from build123d import *

# Parameters (mm, degrees)
F0_W          = 152.4
F0_H          = 203.2
F1_DEPTH      = 6.35
F3_DEPTH      = 63.5
F4_T          = 5
F4_T3_DEPTH   = 73.5
F4_T5_DEPTH   = 137
F6_R          = 13.716
F7_DEPTH      = 76.2
F5_W          = 101.6
F5_H          = 20
F8_DEPTH      = 63.501
F8_DEPTH_BACK = 139.701
F10_DEPTH     = 71.337


# Not quite as in the source:
# - a shell that OpenCascade refuses in one call is made with other operations: the cavity is built on its own and cut out


with BuildPart() as f1:
    # F0 (on Top) → F1 (new body)
    with BuildSketch(Plane.XY):
        Rectangle(F0_W, F0_H)
    extrude(amount=-F1_DEPTH)

    # F2 (on Right) → F3 (join, symmetric)
    with BuildSketch(Plane.YZ):
        Polygon((-101.6, 60), (-101.6, 0), (-38.1, 0), (-38.1, 20), (-68.58, 60), align=None)
    extrude(amount=F3_DEPTH, both=True)

    # F4: shell of thickness 5, made by hand


with BuildPart() as f4_core1:
    # F4_t2: copy of F1
    add(f1.part)

    # the walls: a layer under each face that stays
    f4_faces = [f4_core1.faces().sort_by_distance(p)[0] for p in [
        (0, 101.6, -3.175),
        (76.2, 0, -3.175),
        (-76.2, 0, -3.175),
        (0, 0, 0),
        (0, 0, -6.35),
        (63.5, -69.85, 30),
        (0, -38.1, 10),
        (-63.5, -69.85, 30),
        (0, -53.34, 40),
        (0, -85.09, 60),
    ]]
    thicken(f4_faces, amount=-F4_T, mode=Mode.SUBTRACT)

    # F4_s4 → F4_t3 (cut)
    with BuildSketch(Plane.XZ.offset(33.1)):
        Polygon((63.55, 0.05), (63.5, -5), (58.5, -5), (58.5, 0), align=None)
        Polygon((-63.55, 0.05), (-63.5, -5), (-58.5, -5), (-58.5, 0), align=None)
    extrude(amount=F4_T3_DEPTH, mode=Mode.SUBTRACT)

    # F4_s6 → F4_t5 (cut)
    with BuildSketch(Plane.YZ.offset(-68.5)):
        Polygon((-38.05, 0.05), (-38.1, -5), (-43.1, -5), (-43.1, 0), align=None)
    extrude(amount=F4_T5_DEPTH, mode=Mode.SUBTRACT)


with BuildPart() as f1_1:
    add(f1.part)

    # what is left inside the walls is the cavity
    f4_cavity = [f4_core1.part.solids().sort_by_distance(p)[0] for p in [
        (0, -82.1, -1.3),
    ]]
    add(f4_cavity, mode=Mode.SUBTRACT)

    # F6 (on Right) → F7 (join, symmetric)
    with BuildSketch(Plane.YZ):
        with BuildLine():
            Line((30.48, 0), (5.0091754749, 38.1))
            ThreePointArc((5.0091754749, 38.1), (-12.7, 71.336), (-30.4091754749, 38.1))
            Line((-30.4091754749, 38.1), (-38.1, 19.05))
            Line((-38.1, 19.05), (-38.1, 0))
            Line((-38.1, 0), (-22.9313431488, 0))
            Line((-22.9313431488, 0), (-11.3591754749, 28.664))
            Line((-11.3591754749, 28.664), (-7.7326171703, 28.664))
            Line((-7.7326171703, 28.664), (11.43, 0))
            Line((11.43, 0), (30.48, 0))
        make_face()
        with Locations((-12.7, 50)):
            Circle(F6_R, mode=Mode.SUBTRACT)
    extrude(amount=F7_DEPTH, both=True)

    # F5 (on face) → F8 (cut, two sides)
    with BuildSketch(Plane(origin=(0, -38.1, 0), x_dir=(-1, 0, 0), z_dir=(0, 1, 0))) as f8_sk:
        with Locations((0, 10)):
            Rectangle(F5_W, F5_H)
    extrude(amount=-F8_DEPTH, mode=Mode.SUBTRACT)
    extrude(f8_sk.sketch, amount=F8_DEPTH_BACK, mode=Mode.SUBTRACT)

    # F9 (on face) → F10 (cut, through all)
    with BuildSketch(Plane.XY):
        Polygon((50.8, 11.43), (50.8, 30.48), (-50.8, 30.48), (-50.8, 11.43), (-50.8, -22.9313431488), (-50.8, -38.1), (50.8, -38.1), (50.8, -22.9313431488), align=None)
    extrude(amount=F10_DEPTH, mode=Mode.SUBTRACT)


solid = f1_1.part
The listing builds one solid part. Answer for the finished solid, in the listing's coordinates (mm). A direction names the side the tool comes from. Round coordinates to 2 decimals unless told otherwise and drop trailing zeros. Write each loop counter-clockwise with the first axis right and the second up, starting at its lowest first coordinate (ties: lowest second). Pieces come first, ordered by that corner, then holes. Notation, with made-up numbers: (29, 29) - (42, 29) arc R27 cw to (42, 48) - close; hole circle Ø10 at (-29.75, 48). An arc over 180 degrees is marked (long way). Use one line per item in the form item = value. Start each with the question number.
Item 1: A cutting plane is placed at D-D (z = 11.5). Write down the section's boundary in (x, y).
Item 2: A cutting plane is placed at B-B (y = -17). Write down the section's boundary in (x, z).
Item 3: Flat-ended cylindrical pins translate along their axes: pin 1 Ø10 at (x, y) = (-72.5, -66) entering from +Z; pin 2 Ø5 at (y, z) = (-43.5, 3) entering from +X; pin 3 Ø4 at (x, z) = (-67.5, 8) entering from -Y; pin 4 Ø24.5 at (y, z) = (-12.7, 50) entering from +X. Find the tip coordinate at first contact, or state that the pin passes through.
Item 4: A cutting plane is placed at A-A (x = -19). Write down the section's boundary in (y, z).
Item 5: A tool of negligible diameter and unlimited length cuts with its end or side. For faces 4 (the flat face through (63.678, -17.226, 14.131)), 5 (the flat face through (1, -86, 55)), 6 (the flat face through (1, -41, 20)), 7 (the flat face through (70, -38.1, 10)), from which of +Z, -Z, +X, -X, +Y, -Y can it reach the whole face along a straight path? Write none if from no direction.
Item 6: Find the intervals of material crossed by line 1 (Y direction, x = 67, z = 50); line 2 (X direction, y = -50, z = 19); line 3 (X direction, y = 3, z = 60.5), in increasing order. Write a range as [from, to].
Item 7: Determine the mould class of faces 1 (the flat face through (-70, -69, 0)), 2 (the flat face through (63.68, -34.2, 28.71)), 3 (the flat face through (-1, 101.6, -3)) for opening direction Z: +Z half, -Z half, draft (parallel to the pull), parting line (faces both ways), or undercut.
Item 8: A cutting plane is placed at C-C (z = 50). Write down the section's boundary in (x, y).
The answers:
q1.outline = (-76.2, -38.1) - (-63.5, -38.1) - (-63.5, -101.6) - (-58.5, -101.6) - (-58.5, -43.1) - (-50.8, -43.1) - (-50.8, -18.29) - (-76.2, -18.29) - close; (-76.2, 3.74) - (-50.8, 3.74) - (-50.8, 22.79) - (-76.2, 22.79) - close; (50.8, -43.1) - (58.5, -43.1) - (58.5, -101.6) - (63.5, -101.6) - (63.5, -38.1) - (76.2, -38.1) - (76.2, -18.29) - (50.8, -18.29) - close; (50.8, 3.74) - (76.2, 3.74) - (76.2, 22.79) - (50.8, 22.79) - close
q2.outline = (-76.2, -6.35) - (76.2, -6.35) - (76.2, 0) - (-76.2, 0) - close; (-76.2, 14.69) - (-50.8, 14.69) - (-50.8, 36.98) - (-76.2, 36.98) - close; (-76.2, 63.02) - (-50.8, 63.02) - (-50.8, 70.9) - (-76.2, 70.9) - close; (50.8, 14.69) - (76.2, 14.69) - (76.2, 36.98) - (50.8, 36.98) - close; (50.8, 63.02) - (76.2, 63.02) - (76.2, 70.9) - (50.8, 70.9) - close
q3.pin_1 = 0
q3.pin_2 = 63.5
q3.pin_3 = -38.1
q3.pin_4 = through
q4.outline = (-101.6, -6.35) - (101.6, -6.35) - (101.6, 0) - (-43.1, 0) - (-43.1, -1.35) - (-101.6, -1.35) - close; (-101.6, 55) - (-71.06, 55) - (-44.39, 20) - (-38.1, 20) - (-68.58, 60) - (-101.6, 60) - close
q5.face_4 = +X, -X
q5.face_5 = -Y
q5.face_6 = +Y, -Y
q5.face_7 = +Z, +X, -Y
q6.line_1 = [-34.04, -26.42], [1.02, 8.64]
q6.line_2 = [-63.5, -58.5], [58.5, 63.5]
q6.line_3 = [-76.2, -50.8], [50.8, 76.2]
q7.face_1 = +Z half
q7.face_2 = undercut
q7.face_3 = draft
q8.outline = (-76.2, -34.04) - (-50.8, -34.04) - (-50.8, -26.42) - (-76.2, -26.42) - close; (-76.2, 1.02) - (-50.8, 1.02) - (-50.8, 8.64) - (-76.2, 8.64) - close; (-63.5, -101.6) - (-58.5, -101.6) - (-58.5, -67.25) - (58.5, -67.25) - (58.5, -101.6) - (63.5, -101.6) - (63.5, -60.96) - (-63.5, -60.96) - close; (50.8, -34.04) - (76.2, -34.04) - (76.2, -26.42) - (50.8, -26.42) - close; (50.8, 1.02) - (76.2, 1.02) - (76.2, 8.64) - (50.8, 8.64) - close
